The listing builds one solid part. Answer for the finished solid, in the listing's coordinates (mm). A direction names the side the tool comes from. Coordinates: 2 decimals unless noted, no trailing zeros. Write each loop counter-clockwise with the first axis right and the second up, starting at its lowest first coordinate (ties: lowest second). Pieces come first, ordered by that corner, then holes.
Autodesk Inventor part; units mm, degrees
ref_plane "YZ Plane" through (0, 0, 0) normal (1, 0, 0) x (0, 1, 0)
ref_plane "XZ Plane" through (0, 0, 0) normal (0, 1, 0) x (-1, 0, 0)
ref_plane "XY Plane" through (0, 0, 0) normal (0, 0, 1) x (1, 0, 0)
sketch "Sketch1" plane through (0, 0, 0) normal (0, 1, 0) x (-1, 0, 0)
  line L0 (20, 37.5) -> (-20, 37.5)
  line L1 (-20, 37.5) -> (-20, -20.5)
  line L2 (-20, -20.5) -> (20, -20.5)
  line L3 (20, -20.5) -> (20, 37.5)
  circle A0 centre (14, -11.05) radius 2
  circle A1 centre (14, 28.95) radius 2
  circle A2 centre (-14, -11.05) radius 2
  circle A3 centre (-14, 28.95) radius 2
  circle A4 centre (0, 0) radius 9.4
  circle A5 centre (0, 0) radius 4
  dimension "d0" = 58
  dimension "d1" = 20.5
  dimension "d2" = 40
  dimension "d3" = 20
  dimension "d4" = 4
  dimension "d5" = 4
  dimension "d6" = 40
  dimension "d7" = 11.05
  dimension "d8" = 4
  dimension "d9" = 4
  dimension "d10" = 28
  dimension "d11" = 40
  dimension "d12" = 28
  dimension "d13" = 6
  dimension "d14" = 6
  dimension "d15" = 6
  dimension "d20" = 18.8
  dimension "d21" = 8
extrude "Extrusion1" add sketch "Sketch1" along normal mid plane 27 contours L3 L2 L1 L0 | A4 | A5
extrude "Extrusion2" add sketch "Sketch1" along normal mid plane 31 contours A0 | A1 | A2 | A3
extrude "Extrusion3" add sketch "Sketch1" along normal mid plane 36 contours A4
extrude "Extrusion4" add sketch "Sketch1" along normal blind 22 contours A5
sketch "Sketch2" plane through (-20, 13.5, 37.5) normal (0, 0, 1) x (1, 0, 0)
  circle A0 centre (20, -13.5) radius 15.5
  dimension "d26" = 31
extrude "Extrusion5" add sketch "Sketch2" along normal blind 57
extrude "Extrusion6" add sketch "Sketch1" against normal blind 18 contours A5
hole "Hole1" at (-14, 0, 28.95) direction (0, 1, 0) diameter 3.242 end through all
hole "Hole2" at (14, 0, 28.95) direction (0, 1, 0) diameter 3.242 end through all
hole "Hole3" at (14, 0, -11.05) direction (0, 1, 0) diameter 3.242 end through all
hole "Hole4" at (-14, 0, -11.05) direction (0, 1, 0) diameter 3.242 end through all
sketch "Sketch5" plane through (0, 22, 0) normal (0, 1, 0) x (1, 0, 0)
  circle A0 centre (0, 0) radius 4
extrude "Extrusion7" add sketch "Sketch5" along normal blind 116
thread "Thread1"
properties part number "Motor_Gearbox"
1. Section A-A on x = 0 is taken. Give the vertices of the cut face in (y, z), then the cut area to 3 significant figures.
Results found:
outline: (-18, -9.4) - (-13.5, -9.4) - (-13.5, -20.5) - (13.5, -20.5) - (13.5, -9.4) - (18, -9.4) - (18, -4) - (138, -4) - (138, 4) - (18, 4) - (18, 9.4) - (13.5, 9.4) - (13.5, 37.5) - (15.5, 37.5) - (15.5, 94.5) - (-15.5, 94.5) - (-15.5, 37.5) - (-13.5, 37.5) - (-13.5, 9.4) - (-18, 9.4) - close
area: 4,460 mm2
2. For a pull along Z with two mould halves and no side action, classify faces 1 (the flat face through (-17, 0, 37.5)), 2 (the flat face through (20, 0, 9)), 3 (the flat face through (-14, 0, -11)) as pulls with the +Z half, pulls with the -Z half, needs draft (parallel to the pull), parting line crosses it, or undercut.
Results found:
face 1: pulls with the +Z half
face 2: needs draft
face 3: undercut
3. Find the intervals of material crossed by L1, parallel to X at y = 10, z = -11; L2, parallel to Z at x = 14, y = 12; L3, parallel to Z at x = 14, y = 5, in increasing order.
Results found:
L1: x = -20 to -15.62, -12.38 to 12.38, 15.62 to 20
L2: z = -20.5 to -12.67, -9.43 to 27.33, 30.57 to 37.5
L3: z = -20.5 to -12.67, -9.43 to 27.33, 30.57 to 94.5
4. Section B-B on z = 28.95 is taken. Give the vertices of the cut face in (x, y).
Results found:
outline: (-20, -13.5) - (-16, -13.5) - (-16, -15.5) - (-12, -15.5) - (-12, -13.5) - (12, -13.5) - (12, -15.5) - (16, -15.5) - (16, -13.5) - (20, -13.5) - (20, 13.5) - (16, 13.5) - (16, 15.5) - (15.62, 15.5) - (15.62, 0) - (12.38, 0) - (12.38, 15.5) - (12, 15.5) - (12, 13.5) - (-12, 13.5) - (-12, 15.5) - (-12.38, 15.5) - (-12.38, 0) - (-15.62, 0) - (-15.62, 15.5) - (-16, 15.5) - (-16, 13.5) - (-20, 13.5) - close
5. Flat-ended cylindrical pins translate along their axes: P1, Ø5, axis at x = 10.5, z = 57, coming from the +Y side; P2, Ø10, axis at x = -15.5, z = 49.5, coming from the +Y side; P3, Ø12, axis at x = -12.5, y = 49.5, coming from the +Z side; P4, Ø10, axis at x = -6, y = 46, coming from the +Z side. Find the tip coordinate at first contact, or state that the pin passes through.
Results found:
P1: stops at y = 13.28
P2: stops at y = 11.4
P3: passes through
P4: stops at z = 3.87
6. Section C-C on y = 4.5 is taken. Give the vertices of the cut face in (x, z).
Results found:
outline: (-20, -20.5) - (20, -20.5) - (20, 37.5) - (14.83, 37.5) - (14.83, 94.5) - (-14.83, 94.5) - (-14.83, 37.5) - (-20, 37.5) - close; hole circle Ø3.24 at (-14, -11.05); hole circle Ø3.24 at (-14, 28.95); hole circle Ø3.24 at (14, -11.05); hole circle Ø3.24 at (14, 28.95)
7. Section D-D on z = 0 is taken. Give the vertices of the cut face in (x, y).
Results found:
outline: (-20, -13.5) - (-9.4, -13.5) - (-9.4, -18) - (9.4, -18) - (9.4, -13.5) - (20, -13.5) - (20, 13.5) - (9.4, 13.5) - (9.4, 18) - (4, 18) - (4, 138) - (-4, 138) - (-4, 18) - (-9.4, 18) - (-9.4, 13.5) - (-20, 13.5) - close
8. A tool of negligible diameter and unlimited length cuts with its end or side. For faces 4 (the cylindrical face through (-2.018, -15.368, 65.601)), 5 (the cylindrical face through (2.038, -15.718, -9.176)), 6 (the cylindrical face through (2.038, 15.718, 9.176)), 7 (the flat face through (0, 0, 94.5)), 8 (the flat face through (0, 138, 0)), from which of +Z, -Z, +X, -X, +Y, -Y can it reach the whole face along a straight path? Write none if from no direction.
Results found:
face 4: +Z
face 5: -Y
face 6: +Y
face 7: +Z, +X, -X, +Y, -Y
face 8: +Z, -Z, +X, -X, +Y
